Check sheet for the modelled part. Datum: model origin and axes. Units: mm. A direction names the side the tool comes from. Round coordinates to 2 decimals unless told otherwise and drop trailing zeros. Write each loop counter-clockwise with the first axis right and the second up, starting at its lowest first coordinate (ties: lowest second). Pieces come first, ordered by that corner, then holes. Notation, with made-up numbers: (-32.75, 13) -> (11.25, 13) arc R24 ccw to (11.25, 43) -> close; hole circle Ø11 at (-33.5, 12). An arc over 180 degrees is marked (long way). Write item = value, one per line.
from build123d import *

# Parameters (mm, degrees)
F1_DEPTH  = 1219.2
F2_SIZE   = 1.5875
F5_W      = 34.925
F5_H      = 12.7
F6_DEPTH  = 1219.201
F9_DEPTH  = 1219.201
F10_W     = 2.38125
F10_H     = 6.35
F11_DEPTH = 1219.2


with BuildPart() as f1:
    # F0 (on Front) → F1 (new body)
    with BuildSketch(Plane.XZ):
        Polygon((0, 1.5875), (0, 0), (10.31875, 0), (10.31875, 1.5875), (7.9375, 1.5875), (7.9375, 11.1125), (14.2875, 11.1125), (14.2875, 12.7), (3.96875, 12.7), (3.96875, 11.1125), (6.35, 11.1125), (6.35, 1.5875), align=None)
    extrude(amount=F1_DEPTH)

    # F2
    f2_edges = [f1.edges().sort_by_distance(p)[0] for p in [
        (6.35, -609.6, 1.5875),
        (7.9375, -609.6, 11.1125),
    ]]
    chamfer(f2_edges, length=F2_SIZE)

    # F3: F1 across face


with BuildPart() as f1_1:
    add(f1.part)
    add(f1.part.mirror(Plane(origin=(14.2875, -609.6, 11.90625), x_dir=(0, 1, 0), z_dir=(1, 0, 0))))

    # F4: F1 across face


with BuildPart() as f1_2:
    add(f1_1.part)
    add(f1_1.part.mirror(Plane(origin=(28.575, -609.6, 0.79375), x_dir=(0, 1, 0), z_dir=(1, 0, 0))))

    # F5 (on face) → F6 (cut, through all)
    with BuildSketch(Plane.XZ.offset(1219.2)):
        with Locations((39.6875, 6.35)):
            Rectangle(F5_W, F5_H)
    extrude(amount=-F6_DEPTH, mode=Mode.SUBTRACT)

    # F7: F1 across face


with BuildPart() as f1_3:
    add(f1_2.part)
    add(f1_2.part.mirror(Plane(origin=(0, -609.6, 0.79375), x_dir=(0, -1, 0), z_dir=(-1, 0, 0))))

    # F8 (on face) → F9 (cut, through all)
    with BuildSketch(Plane.XZ.offset(1219.2)):
        Polygon((7.9375, 12.7), (7.9375, 9.525), (9.525, 11.1125), (19.05, 11.1125), (20.6375, 9.525), (20.6375, 1.5875), (18.25625, 1.5875), (18.25625, 0), (22.225, 0), (22.225, 12.7), align=None)
    extrude(amount=-F9_DEPTH, mode=Mode.SUBTRACT)

    # F10 (on face) → F11 (join, through all)
    with BuildSketch(Plane.XZ.offset(1219.2)):
        Polygon((34.925, 12.7), (7.9375, 12.7), (7.9375, 11.1125), (33.3375, 11.1125), (33.3375, 7.9375), (30.95625, 7.9375), (30.95625, 0), (34.925, 0), align=None)
        with Locations((9.128125, 4.7625)):
            Rectangle(F10_W, F10_H)
    extrude(amount=-F11_DEPTH)


solid = f1_3.part
(1) Go/stop test with a flat-tipped pin: P1, Ø6, axis at x = 15, y = -1063, coming from the -Z side. Record where the tip stops, or that it passes through.
Worked answers:
P1 = 11.11
(2) Sectioned sample at B-B on x = 21. Enter the section's corners in (y, z), then the cut area to 3 significant figures.
Worked answers:
outline = (-1219.2, 11.11) -> (0, 11.11) -> (0, 12.7) -> (-1219.2, 12.7) -> close
area = 1,940 mm²
(3) Access from +Z, -Z, +X, -X, +Y, -Y to the whole of each face (thin tool, end or side, straight path). Record for faces 1 (the flat face through (20, -618, 12.7)), 2 (the flat face through (20, -618, 11.112)).
Worked answers:
face_1 = +Z, +X, -X, +Y, -Y
face_2 = +Y, -Y
(4) Material ranges on L1, parallel to Z at x = 9, y = -555.5; L2, parallel to Z at x = -20, y = -527; L3, parallel to X at y = -1104, z = 0.5 (3 decimals), recorded low to high. Write a range as [from, to].
Worked answers:
L1 = [0, 7.94], [11.11, 12.7]
L2 = [0, 1.59], [10.16, 12.7]
L3 = [-22.225, -18.256], [-10.319, 10.319], [30.956, 34.925]
